from build123d import *

# Parameters (mm, degrees)
MODEL_R             = 1.75
BOSS_EXTRUDE1_DEPTH = 5


with BuildPart() as part:
    # Model → Boss-Extrude1 (new body)
    with BuildSketch(Plane.XY):
        Polygon((5, -152.5), (0, -152.5), (0, -132.5), (5, -132.5), (5, -112.5), (0, -112.5), (0, -92.5), (5, -92.5), (5, -72.5), (0, -72.5), (0, -52.5), (5, -52.5), (5, -32.5), (0, -32.5), (0, -12.5), (5, -12.5), (5, 7.5), (0, 7.5), (0, 27.5), (5, 27.5), (5, 47.5), (0, 47.5), (0, 67.5), (5, 67.5), (5, 87.5), (0, 87.5), (0, 107.5), (5, 107.5), (5, 127.5), (0, 127.5), (0, 147.5), (5, 147.5), (5, 167.5), (-2.5, 167.5), (-2.5, 172.5), (-7.5, 172.5), (-7.5, 167.5), (-15, 167.5), (-15, 147.5), (-10, 147.5), (-10, 127.5), (-15, 127.5), (-15, 107.5), (-10, 107.5), (-10, 87.5), (-15, 87.5), (-15, 67.5), (-10, 67.5), (-10, 47.5), (-15, 47.5), (-15, 27.5), (-10, 27.5), (-10, 7.5), (-15, 7.5), (-15, -12.5), (-10, -12.5), (-10, -32.5), (-15, -32.5), (-15, -52.5), (-10, -52.5), (-10, -72.5), (-15, -72.5), (-15, -92.5), (-10, -92.5), (-10, -112.5), (-15, -112.5), (-15, -132.5), (-10, -132.5), (-10, -152.5), (-15, -152.5), (-15, -172.5), (-7.5, -172.5), (-7.5, -177.5), (-2.5, -177.5), (-2.5, -172.5), (5, -172.5), align=None)
        with Locations((-5, 142.5)):
            Circle(MODEL_R, mode=Mode.SUBTRACT)
        with Locations((-5, 117.5)):
            Circle(MODEL_R, mode=Mode.SUBTRACT)
        with Locations((-5, 92.5)):
            Circle(MODEL_R, mode=Mode.SUBTRACT)
        with Locations((-5, 67.5)):
            Circle(MODEL_R, mode=Mode.SUBTRACT)
        with Locations((-5, 42.5)):
            Circle(MODEL_R, mode=Mode.SUBTRACT)
        with Locations((-5, 17.5)):
            Circle(MODEL_R, mode=Mode.SUBTRACT)
        with Locations((-5, -7.5)):
            Circle(MODEL_R, mode=Mode.SUBTRACT)
        with Locations((-5, -32.5)):
            Circle(MODEL_R, mode=Mode.SUBTRACT)
        with Locations((-5, -57.5)):
            Circle(MODEL_R, mode=Mode.SUBTRACT)
        with Locations((-5, -82.5)):
            Circle(MODEL_R, mode=Mode.SUBTRACT)
        with Locations((-5, -107.5)):
            Circle(MODEL_R, mode=Mode.SUBTRACT)
        with Locations((-5, -132.5)):
            Circle(MODEL_R, mode=Mode.SUBTRACT)
        with Locations((-5, -157.5)):
            Circle(MODEL_R, mode=Mode.SUBTRACT)
    extrude(amount=BOSS_EXTRUDE1_DEPTH)


solid = part.part
Verification items for the finished model (mm, model axes). Coordinates: 2 decimals unless noted, no trailing zeros. Order: outer loops, then holes, each group sorted by start corner. A loop starts at its lowest first (then second) coordinate and runs counter-clockwise, first axis right, second up. Notation, with made-up numbers: M -6.75,-7 L 42.25,-7 A22 ccw 42.25,17 Z; hole C 66.25,50 d8. An arc over 180 degrees is marked long. One line per item, written item: value. Start each with the question number.
Item 1: Sectioned sample at A-A (z = 2.6). Count the separate pieces of the cut face and the enclosed holes in it, then the cut area to 3 significant figures.
Item 2: Gauge pin test, flat ends, axial feed: pin 1 (3 mm diameter, centred on y = 11, z = 2, fed in from +X); pin 2 (2.5 mm diameter, centred on x = -13, z = 2.5, fed in from -Y); pin 3 (2.5 mm diameter, centred on x = 3.5, z = 3, fed in from +Y); pin 4 (2 mm diameter, centred on x = -5, y = -157.5, fed in from -Z). Record the tip position at first contact, or that the pin passes through.
Item 3: Scan lines: probe 1 along X at (y, z) = (-157.5, 2.3); probe 2 along X at (y, z) = (92.5, 1.7); probe 3 along X at (y, z) = (104.5, 2.8). Record each from-to range of solid material in increasing order.
Item 4: Sectioned sample at B-B (y = 130.5). Enter the section's corners in (x, z).
Conclusion:
1. separate pieces: 1
1. enclosed holes: 13
1. area: 5,120 mm^2
2. pin 1: stops at x = 0
2. pin 2: stops at y = -172.5
2. pin 3: stops at y = 167.5
2. pin 4: passes through
3. probe 1: x = -15 to -6.75, -3.25 to 5
3. probe 2: x = -10 to -6.75, -3.25 to 0
3. probe 3: x = -10 to 0
4. outline: M -10,0 L 0,0 L 0,5 L -10,5 Z
